Could you check a few things on this model? Use its own coordinates, in mm. Give positions to 0.01 mm unless a question says otherwise; leave off trailing zeros. Answer as CSV lines item,"result". Start each with the question number.
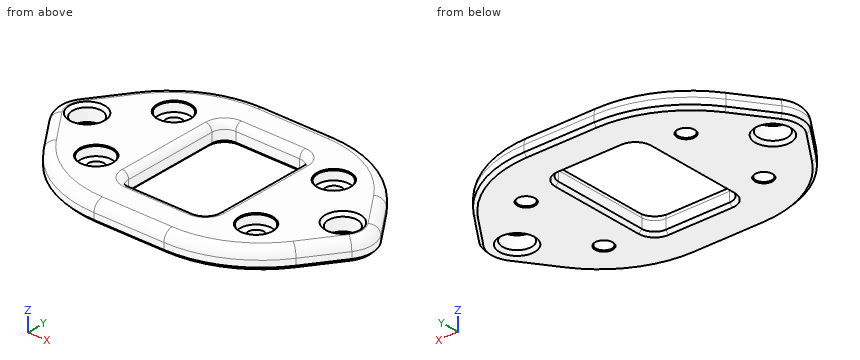
from build123d import *

# Parameters (mm, degrees)
F0_R     = 2.5
F0_R_2   = 4.5
F1_DEPTH = 6
F2_R     = 5
F3_DEPTH = 3
F4_R     = 3
F5_SIZE  = 1
F6_SIZE  = 1
F7_SIZE  = 1
F8_SIZE  = 0.25
F9_R     = 2


with BuildPart() as f1:
    # F0 (on Top) → F1 (new body)
    with BuildSketch(Plane.XY):
        with BuildLine():
            Line((-10.920631, -31), (0, -31))
            Line((0, -31), (10.920631, -31))
            ThreePointArc((10.920631, -31), (26.983553, -27.096343), (39.463381, -16.256145))
            Line((39.463381, -16.256145), (47.303487, -5.208723))
            ThreePointArc((47.303487, -5.208723), (48.963923, 0), (47.303487, 5.208723))
            Line((47.303487, 5.208723), (39.463381, 16.256145))
            ThreePointArc((39.463381, 16.256145), (26.983553, 27.096343), (10.920631, 31))
            Line((10.920631, 31), (0, 31))
            Line((0, 31), (-10.920631, 31))
            ThreePointArc((-10.920631, 31), (-26.983553, 27.096343), (-39.463381, 16.256145))
            Line((-39.463381, 16.256145), (-47.303487, 5.208723))
            ThreePointArc((-47.303487, 5.208723), (-48.963923, 0), (-47.303487, -5.208723))
            Line((-47.303487, -5.208723), (-39.463381, -16.256145))
            ThreePointArc((-39.463381, -16.256145), (-26.983553, -27.096343), (-10.920631, -31))
        make_face()
        with Locations((-25, -14)):
            Circle(F0_R, mode=Mode.SUBTRACT)
        with Locations((25, -14)):
            Circle(F0_R, mode=Mode.SUBTRACT)
        with Locations((-40, 0)):
            Circle(F0_R_2, mode=Mode.SUBTRACT)
        with Locations((-25, 14)):
            Circle(F0_R, mode=Mode.SUBTRACT)
        with BuildLine():
            Line((-10, 19), (0, 19))
            Line((0, 19), (10, 19))
            ThreePointArc((10, 19), (12.828427, 17.828427), (14, 15))
            Line((14, 15), (14, 10))
            Line((14, 10), (14, -10))
            Line((14, -10), (14, -15))
            ThreePointArc((14, -15), (12.828427, -17.828427), (10, -19))
            Line((10, -19), (0, -19))
            Line((0, -19), (-10, -19))
            ThreePointArc((-10, -19), (-12.828427, -17.828427), (-14, -15))
            Line((-14, -15), (-14, -10))
            Line((-14, -10), (-14, 10))
            Line((-14, 10), (-14, 15))
            ThreePointArc((-14, 15), (-12.828427, 17.828427), (-10, 19))
        make_face(mode=Mode.SUBTRACT)
        with Locations((40, 0)):
            Circle(F0_R_2, mode=Mode.SUBTRACT)
        with Locations((25, 14)):
            Circle(F0_R, mode=Mode.SUBTRACT)
    extrude(amount=F1_DEPTH)

    # F2 (on face) → F3 (cut)
    with BuildSketch(Plane.XY.offset(6)):
        with Locations((-25, 14)):
            Circle(F2_R)
        with Locations((25, 14)):
            Circle(F2_R)
        with Locations((25, -14)):
            Circle(F2_R)
        with Locations((-25, -14)):
            Circle(F2_R)
    extrude(amount=-F3_DEPTH, mode=Mode.SUBTRACT)

    # F4
    f4_edges = [f1.edges().sort_by_distance(p)[0] for p in [
        (0, 31, 6),
    ]]
    fillet(f4_edges, radius=F4_R)

    # F5
    f5_edges = [f1.edges().sort_by_distance(p)[0] for p in [
        (26.983553, -27.096343, 0),
    ]]
    chamfer(f5_edges, length=F5_SIZE)

    # F6
    f6_edges = [f1.edges().sort_by_distance(p)[0] for p in [
        (-14, 0, 0),
    ]]
    chamfer(f6_edges, length=F6_SIZE)

    # F7
    f7_edges = [f1.edges().sort_by_distance(p)[0] for p in [
        (-44.5, 0, 6),
        (35.5, 0, 6),
        (35.5, 0, 0),
        (-44.5, 0, 0),
    ]]
    chamfer(f7_edges, length=F7_SIZE)

    # F8
    f8_edges = [f1.edges().sort_by_distance(p)[0] for p in [
        (-30, -14, 6),
        (-30, 14, 6),
        (20, 14, 6),
        (20, -14, 6),
        (22.5, -14, 0),
        (22.5, 14, 0),
        (-27.5, 14, 0),
        (-27.5, -14, 0),
    ]]
    chamfer(f8_edges, length=F8_SIZE)

    # F9
    f9_edges = [f1.edges().sort_by_distance(p)[0] for p in [
        (0, 19, 6),
    ]]
    fillet(f9_edges, radius=F9_R)


solid = f1.part
1. Imagine slicing it at A-A, the plane y = 0. State how many separate pieces and enclosed holes the cut face has, plus the area to 3 significant figures.
2. Will these pins go through, and if not, where does the flat tip stop? P1, Ø1, axis at y = -15.5, z = 2, coming from the +X side; P2, Ø5.5, axis at x = -40, y = 0, coming from the -Z side; P3, Ø1.5, axis at y = -7, z = 2.5, coming from the -X side; P4, Ø8, axis at x = 25, y = -14, coming from the +Z side.
3. Please list where these lines run through material, in increasing order: line 1 (Y direction, x = 6.5, z = 1.5); line 2 (X direction, y = 18, z = 3.75); line 3 (Y direction, x = -25, z = 1.8).
Solutions:
1,separate pieces,"4"
1,enclosed holes,"0"
1,area,"300 mm²"
2,P1,"x = 40.35"
2,P2,"through"
2,P3,"x = -46.56"
2,P4,"z = 3"
3,line 1,"-31 to -19, 19 to 31"
3,line 2,"-38.02 to -28, -22 to -12.65, 12.65 to 22, 28 to 38.02"
3,line 3,"-28.04 to -16.5, -11.5 to 11.5, 16.5 to 28.04"
